The listing builds one solid part. Answer for the finished solid, in the listing's coordinates (mm). A direction names the side the tool comes from. Coordinates: 2 decimals unless noted, no trailing zeros. Order: outer loops, then holes, each group sorted by start corner. A loop starts at its lowest first (then second) coordinate and runs counter-clockwise, first axis right, second up. Notation, with made-up numbers: M 53.5,85 L 67.5,85 A14 ccw 67.5,89 Z; hole C 73.25,-24 d2. An arc over 180 degrees is marked long. One line per item, written item: value. Start each with the question number.
Q1. The part is cut by section A-A on x = 0. Give the vertices of the cut face in (y, z).
Q2. Determine the mould class of faces 3 (the flat face through (-12.5, -1, 25)), 4 (the flat face through (0, -62.5, 25)), 5 (the flat face through (2.4, 52.4, 10)) for opening direction Y: pulls with the +Y half, pulls with the -Y half, needs draft (parallel to the pull), parting line crosses it, or undercut.
Q3. Straight lines are drawn through the part: line 1 along Y through (x, z) = (0, 2.75); line 2 along Y through (x, z) = (0, 21); line 3 along X through (y, z) = (-50, 7). For each, find the intervals that lie inside material, in ascending order. Write a range as [from, to].
Q4. The part is cut by section B-B on z = 22. Give the vertices of the cut face in (x, y).
Q5. The part is cut by section C-C on y = 50. Give the vertices of the cut face in (x, z), then the cut area to 3 significant figures.
Q6. Each of these flat-tipped pins is pushed along its axis until it touches: pin 1 Ø12 at (x, y) = (-2, 35) entering from -Z; pin 2 Ø3.5 at (x, y) = (2.5, 1.5) entering from -Z. Where does it stop, or does it pass through?
Q7. For faces 1 (the flat face through (2.4, -47.6, 10)), 2 (the flat face through (0, 62.5, 25)), determine the directions among +Z, -Z, +X, -X, +Y, -Y from which every point of the face is accessible in a straight line to the end or side of a thin tool.
```python
from build123d import *

# Parameters (mm, degrees)
F0_W           = 25
F0_H           = 125
F1_DEPTH       = 50
F3_D           = 6.4
F3_CBORE_D     = 11
F3_CBORE_DEPTH = 10


with BuildPart() as f1:
    # F0 (on Top) → F1 (new body)
    with BuildSketch(Plane.XY):
        Rectangle(F0_W, F0_H)
    extrude(amount=F1_DEPTH)

    # F3 (through all)
    with Locations(Plane(origin=(0, 0, 0), x_dir=(1, 0, 0), z_dir=(0, 0, -1))):
        with Locations((0, 50), (0, -50), (0, 0)):
            CounterBoreHole(F3_D / 2, F3_CBORE_D / 2, F3_CBORE_DEPTH)


solid = f1.part
```
Output:
1. outline: M -62.5,0 L -55.5,0 L -55.5,10 L -53.2,10 L -53.2,50 L -62.5,50 Z; M -46.8,10 L -44.5,10 L -44.5,0 L -5.5,0 L -5.5,10 L -3.2,10 L -3.2,50 L -46.8,50 Z; M 3.2,10 L 5.5,10 L 5.5,0 L 44.5,0 L 44.5,10 L 46.8,10 L 46.8,50 L 3.2,50 Z; M 53.2,10 L 55.5,10 L 55.5,0 L 62.5,0 L 62.5,50 L 53.2,50 Z
2. face 3: needs draft
2. face 4: pulls with the -Y half
2. face 5: undercut
3. line 1: y = [-62.5, -55.5], [-44.5, -5.5], [5.5, 44.5], [55.5, 62.5]
3. line 2: y = [-62.5, -53.2], [-46.8, -3.2], [3.2, 46.8], [53.2, 62.5]
3. line 3: x = [-12.5, -5.5], [5.5, 12.5]
4. outline: M -12.5,-62.5 L 12.5,-62.5 L 12.5,62.5 L -12.5,62.5 Z; hole C 0,-50 d6.4; hole C 0,0 d6.4; hole C 0,50 d6.4
5. outline: M -12.5,0 L -5.5,0 L -5.5,10 L -3.2,10 L -3.2,50 L -12.5,50 Z; M 3.2,10 L 5.5,10 L 5.5,0 L 12.5,0 L 12.5,50 L 3.2,50 Z
5. area: 884 mm^2
6. pin 1: stops at z = 0
6. pin 2: stops at z = 10
7. face 1: -Z
7. face 2: +Z, -Z, +X, -X, +Y
